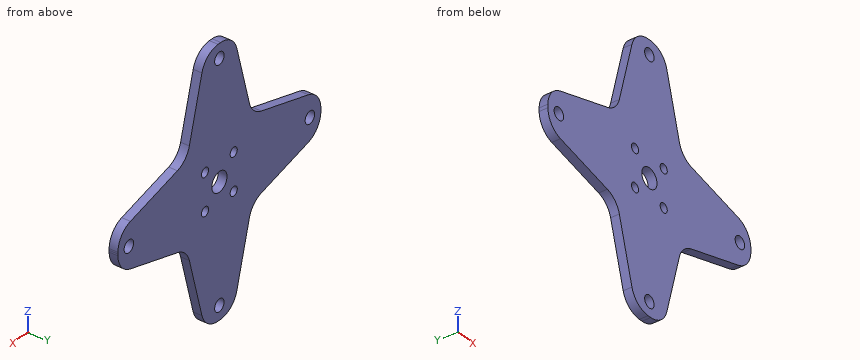
```python
from build123d import *

# Parameters (mm, degrees)
SKETCH_1_R      = 2.8
SKETCH_1_R_2    = 2.1
SKETCH_1_R_3    = 4.5
EXTRUDE_1_DEPTH = 4
FILLET_1_R      = 10


with BuildPart() as part:
    # 草图1 → 凸台-拉伸1 (new body)
    # profile 1 of 5: a face of its own
    with BuildSketch(Plane(origin=(0, 0, 0), x_dir=(1, 0, 0), z_dir=(0, 1, 0))):
        with BuildLine():
            Line((-24.400651417, 0), (-19.24418704, 19.24418704))
            Line((-19.24418704, 19.24418704), (-59.39696962, 8.485281374))
            ThreePointArc((-59.39696962, 8.485281374), (-60, 0), (-59.39696962, -8.485281374))
            Line((-59.39696962, -8.485281374), (-19.24418704, -19.24418704))
            Line((-19.24418704, -19.24418704), (-24.400651417, 0))
        make_face()
        with Locations(Location((-53.5, 0, 0), (0, 0, 270))):
            Circle(SKETCH_1_R, mode=Mode.SUBTRACT)
    # profile 2 of 5: a face of its own
    with BuildSketch(Plane(origin=(0, 0, 0), x_dir=(1, 0, 0), z_dir=(0, 1, 0))):
        Polygon((24.400651417, 0), (19.24418704, 19.24418704), (0, 24.400651417), (-19.24418704, 19.24418704), (-24.400651417, 0), (-19.24418704, -19.24418704), (0, -24.400651417), (19.24418704, -19.24418704), align=None)
        with Locations(Location((-8.485281374, -8.485281374, 0), (0, 0, 270))):
            Circle(SKETCH_1_R_2, mode=Mode.SUBTRACT)
        with Locations(Location((0, 0, 0), (0, 0, 270))):
            Circle(SKETCH_1_R_3, mode=Mode.SUBTRACT)
        with Locations(Location((8.485281374, -8.485281374, 0), (0, 0, 270))):
            Circle(SKETCH_1_R_2, mode=Mode.SUBTRACT)
        with Locations(Location((-8.485281374, 8.485281374, 0), (0, 0, 270))):
            Circle(SKETCH_1_R_2, mode=Mode.SUBTRACT)
        with Locations(Location((8.485281374, 8.485281374, 0), (0, 0, 270))):
            Circle(SKETCH_1_R_2, mode=Mode.SUBTRACT)
    # profile 3 of 5: a face of its own
    with BuildSketch(Plane(origin=(0, 0, 0), x_dir=(1, 0, 0), z_dir=(0, 1, 0))):
        with BuildLine():
            Line((19.24418704, 19.24418704), (8.485281374, 59.39696962))
            ThreePointArc((8.485281374, 59.39696962), (0, 60), (-8.485281374, 59.39696962))
            Line((-8.485281374, 59.39696962), (-19.24418704, 19.24418704))
            Line((-19.24418704, 19.24418704), (0, 24.400651417))
            Line((0, 24.400651417), (19.24418704, 19.24418704))
        make_face()
        with Locations(Location((0, 53.5, 0), (0, 0, 270))):
            Circle(SKETCH_1_R, mode=Mode.SUBTRACT)
    # profile 4 of 5: a face of its own
    with BuildSketch(Plane(origin=(0, 0, 0), x_dir=(1, 0, 0), z_dir=(0, 1, 0))):
        with BuildLine():
            Line((59.39696962, 8.485281374), (19.24418704, 19.24418704))
            Line((19.24418704, 19.24418704), (24.400651417, 0))
            Line((24.400651417, 0), (19.24418704, -19.24418704))
            Line((19.24418704, -19.24418704), (59.39696962, -8.485281374))
            ThreePointArc((59.39696962, -8.485281374), (59.849052529, -4.253341205), (60, 0))
            ThreePointArc((60, 0), (59.849052529, 4.253341205), (59.39696962, 8.485281374))
        make_face()
        with Locations(Location((53.5, 0, 0), (0, 0, 270))):
            Circle(SKETCH_1_R, mode=Mode.SUBTRACT)
    # profile 5 of 5: a face of its own
    with BuildSketch(Plane(origin=(0, 0, 0), x_dir=(1, 0, 0), z_dir=(0, 1, 0))):
        with BuildLine():
            Line((8.485281374, -59.39696962), (19.24418704, -19.24418704))
            Line((19.24418704, -19.24418704), (0, -24.400651417))
            Line((0, -24.400651417), (-19.24418704, -19.24418704))
            Line((-19.24418704, -19.24418704), (-8.485281374, -59.39696962))
            ThreePointArc((-8.485281374, -59.39696962), (0, -60), (8.485281374, -59.39696962))
        make_face()
        with Locations(Location((0, -53.5, 0), (0, 0, 270))):
            Circle(SKETCH_1_R, mode=Mode.SUBTRACT)
    extrude(amount=EXTRUDE_1_DEPTH)

    # 圆角1
    fillet_1_edges = [part.edges().sort_by_distance(p)[0] for p in [
        (-19.24418704, 2, -19.24418704),
        (-8.485281374, 2, -59.39696962),
        (8.485281374, 2, -59.39696962),
        (19.24418704, 2, -19.24418704),
        (59.39696962, 2, -8.485281374),
        (59.39696962, 2, 8.485281374),
        (19.24418704, 2, 19.24418704),
        (8.485281374, 2, 59.39696962),
        (-8.485281374, 2, 59.39696962),
        (-19.24418704, 2, 19.24418704),
        (-59.39696962, 2, 8.485281374),
        (-59.39696962, 2, -8.485281374),
    ]]
    fillet(fillet_1_edges, radius=FILLET_1_R)


solid = part.part
```
Check sheet for the modelled part. Datum: model origin and axes. Units: mm. Round coordinates to 2 decimals unless told otherwise and drop trailing zeros. Order: outer loops, then holes, each group sorted by start corner. A loop starts at its lowest first (then second) coordinate and runs counter-clockwise, first axis right, second up.
1) Section check C-C (z = -33.5). Record the boundary of the cut face in (x, y), and give its area (3 significant figures).
2) Section check A-A (y = 0.8). Give the number of separate pieces and of enclosed holes in the cut face, and give its area (3 significant figures).
3) Go/stop test with a flat-tipped pin: pin 1 Ø5 at (x, z) = (-53.5, 0) entering from +Y. Record where the tip stops, or that it passes through.
4) Scan lines: line 1 (Z direction, x = -8.5, y = 2.7); line 2 (Z direction, x = 0.5, y = 0.2) (3 decimals); line 3 (X direction, y = 1.1, z = 9.5). Record each from-to range of solid material in increasing order.
5) Section check B-B (x = 12). Record the boundary of the cut face in (y, z).
Result:
1. outline: (-15.42, 0) - (15.42, 0) - (15.42, 4) - (-15.42, 4) - close
1. area: 123 mm2
2. separate pieces: 1
2. enclosed holes: 9
2. area: 5,690 mm2
3. pin 1: passes through
4. line 1: z = -56.19 to -10.59, -6.39 to 6.39, 10.59 to 56.19
4. line 2: z = -59.998 to -56.255, -50.745 to -4.472, 4.472 to 50.745, 56.255 to 59.998
4. line 3: x = -54.65 to -10.32, -6.65 to 6.65, 10.32 to 54.65
5. outline: (0, -46.28) - (4, -46.28) - (4, 46.28) - (0, 46.28) - close
